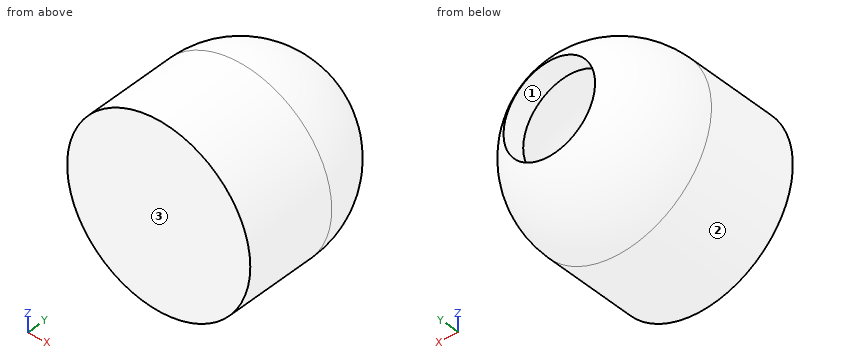
from build123d import *

# Parameters (mm, degrees)
SKETCH3_R          = 2.5
CUT_EXTRUDE1_DEPTH = 3


with BuildPart() as part:
    # Sketch1 → Revolve2 (revolve)
    with BuildSketch(Plane.XY):
        with BuildLine():
            ThreePointArc((0, -5), (5, 0), (0, 5))
            Line((0, 5), (0, -5))
        make_face()
        with BuildLine():
            ThreePointArc((5, 0), (3.535533906, -3.535533906), (0, -5))
            Line((0, -5), (5, -5))
            Line((5, -5), (5, 0))
        make_face()
    revolve(axis=Axis((0, 5, 0), (0, -1, 0)))

    # Sketch2 → Cut-Revolve1 (revolve, cut)
    with BuildSketch(Plane.XY):
        with BuildLine():
            Line((0, 4), (0, -4))
            ThreePointArc((0, -4), (4, 0), (0, 4))
        make_face()
    revolve(axis=Axis((0, 4, 0), (0, -1, 0)), mode=Mode.SUBTRACT)

    # Sketch3 → Cut-Extrude1 (cut)
    with BuildSketch(Plane(origin=(0, 5, 0), x_dir=(1, 0, 0), z_dir=(0, 1, 0))):
        with Locations(Location((0, 0, 0), (0, 0, 90))):
            Circle(SKETCH3_R)
    extrude(amount=-CUT_EXTRUDE1_DEPTH, mode=Mode.SUBTRACT)


solid = part.part
Part model, mm, in its own coordinate system. Face numbers are marked on the shaded views. Coordinates: 2 decimals unless noted, no trailing zeros. Order: outer loops, then holes, each group sorted by start corner. A loop starts at its lowest first (then second) coordinate and runs counter-clockwise, first axis right, second up. Notation, with made-up numbers: (-26, -27.5) - (26, -27.5) arc R23 ccw to (26, 11.5) - close; hole circle Ø9 at (30, 46). An arc over 180 degrees is marked (long way). Use CSV: the item, a comma, the result in double quotes.
Item 1: Probe probe 1 along X at (y, z) = (3.9, 0); probe 2 along X at (y, z) = (3.65, 0); probe 3 along Z at (x, y) = (3, -1). List the from-to ranges inside material, lowest first.
Solved:
probe 1,"x = -3.13 to -2.5, 2.5 to 3.13"
probe 2,"x = -3.42 to -2.5, 2.5 to 3.42"
probe 3,"z = -4 to -2.45, 2.45 to 4"
Item 2: Saw through at A-A on x = 0. Give the cut face in (y, z).
Solved:
outline,"(-5, -5) - (0, -5) arc R5 ccw to (4.33, -2.5) - (3.12, -2.5) arc R4 cw (long way) to (3.12, 2.5) - (4.33, 2.5) arc R5 ccw to (0, 5) - (-5, 5) - close"
Item 3: Saw through at D-D on y = 0.5. Give the cut face in (x, z).
Solved:
outline,"circle Ø9.95 at (0, 0); hole circle Ø7.94 at (0, 0)"
Item 4: Mould opens along X. For the marked faces 1, 2 and 3 say: +X half, -X half, draft (parallel to the pull), parting line (faces both ways), or undercut.
Solved:
face 1,"undercut"
face 2,"parting line"
face 3,"draft"
Item 5: Drop flat-ended pins along their axis: P1, Ø2, axis at y = -0.5, z = -3.5, coming from the +X side; P2, Ø3, axis at y = 1.5, z = -0.5, coming from the -X side; P3, Ø2, axis at y = 2.5, z = -0.5, coming from the +X side. Give the stop position or say it passes through.
Solved:
P1,"stops at x = 4.33"
P2,"stops at x = -5"
P3,"stops at x = 4.75"
Item 6: Saw through at C-C on y = -3. Give the cut face in (x, z).
Solved:
outline,"circle Ø10 at (0, 0); hole circle Ø5.29 at (0, 0)"
Item 7: Saw through at B-B on z = 0. Give the cut face in (x, y), and give its area (3 significant figures).
Solved:
outline,"(-5, -5) - (5, -5) - (5, 0) arc R5 ccw to (2.5, 4.33) - (2.5, 3.12) arc R4 cw (long way) to (-2.5, 3.12) - (-2.5, 4.33) arc R5 ccw to (-5, 0) - close"
area,"33.7 mm²"
